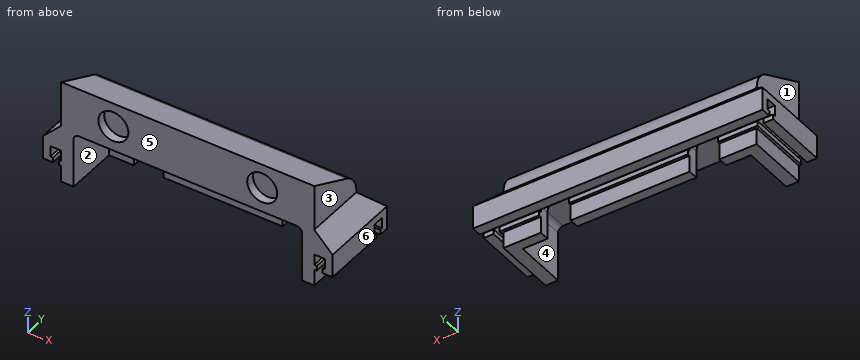
```python
from build123d import *

# Parameters (mm, degrees)
SKETCH1_W           = 102
SKETCH1_H           = 30
BOSS_EXTRUDE1_DEPTH = 25
CUT_EXTRUDE1_DEPTH  = 21
BOSS_EXTRUDE2_DEPTH = 102
SKETCH4_R           = 6.05
CUT_EXTRUDE2_DEPTH  = 3.5
FILLET1_R           = 10
CUT_EXTRUDE3_DEPTH  = 23.5
SKETCH6_W           = 1
SKETCH6_H           = 2
BOSS_EXTRUDE3_DEPTH = 25
SKETCH7_W           = 2
SKETCH7_H           = 1
BOSS_EXTRUDE4_DEPTH = 116.7
CUT_EXTRUDE4_DEPTH  = 7.35
SKETCH9_W           = 2.35
SKETCH9_H           = 1
SKETCH9_W_2         = 12
CUT_EXTRUDE5_DEPTH  = 3


with BuildPart() as part:
    # Sketch1 → Boss-Extrude1 (new body)
    with BuildSketch(Plane(origin=(0, 0, 0), x_dir=(1, 0, 0), z_dir=(0, 1, 0))):
        Rectangle(SKETCH1_W, SKETCH1_H)
    extrude(amount=BOSS_EXTRUDE1_DEPTH)

    # Sketch2 → Cut-Extrude1 (cut)
    with BuildSketch(Plane.XZ):
        with BuildLine():
            Line((-46, -37), (46, -37))
            Line((46, -37), (46, 5))
            ThreePointArc((46, 5), (45.414213562, 6.414213562), (44, 7))
            Line((44, 7), (-44, 7))
            ThreePointArc((-44, 7), (-45.414213562, 6.414213562), (-46, 5))
            Line((-46, 5), (-46, -37))
        make_face()
    extrude(amount=-CUT_EXTRUDE1_DEPTH, mode=Mode.SUBTRACT)

    # Sketch3 → Boss-Extrude2 (add)
    with BuildSketch(Plane(origin=(51, 0, 0), x_dir=(0, 0, -1), z_dir=(1, 0, 0))):
        Polygon((-15, 25), (-26.657691454, 0), (-15, 0), align=None)
    extrude(amount=-BOSS_EXTRUDE2_DEPTH)

    # Sketch4 → Cut-Extrude2 (cut)
    with BuildSketch(Plane.XZ):
        with Locations(Location((-30, 17, 0), (0, 0, 270))):
            Circle(SKETCH4_R)
        with Locations(Location((30, 17, 0), (0, 0, 270))):
            Circle(SKETCH4_R)
    extrude(amount=-CUT_EXTRUDE2_DEPTH, mode=Mode.SUBTRACT)

    # Fillet1
    fillet1_edges = [part.edges().sort_by_distance(p)[0] for p in [
        (0, 25, 15),
    ]]
    fillet(fillet1_edges, radius=FILLET1_R)

    # Sketch5 → Cut-Extrude3 (cut)
    with BuildSketch(Plane(origin=(0, 25, 0), x_dir=(1, 0, 0), z_dir=(0, 1, 0))):
        with BuildLine():
            Line((-24, 26), (-24, 4))
            ThreePointArc((-24, 4), (-30, -2), (-36, 4))
            Line((-36, 4), (-36, 26))
            ThreePointArc((-36, 26), (-30, 32), (-24, 26))
        make_face()
        with BuildLine():
            Line((24, 4), (24, 26))
            ThreePointArc((24, 26), (30, 32), (36, 26))
            Line((36, 26), (36, 4))
            ThreePointArc((36, 4), (30, -2), (24, 4))
        make_face()
    extrude(amount=-CUT_EXTRUDE3_DEPTH, mode=Mode.SUBTRACT)

    # Sketch6 → Boss-Extrude3 (add)
    with BuildSketch(Plane.XZ):
        Polygon((51, -2), (55.35, -2), (55.35, -6.35), (54.35, -6.35), (54.35, -8.35), (58.35, -8.35), (58.35, 1), (51, 8.35), align=None)
        with Locations((51.5, -7.35)):
            Rectangle(SKETCH6_W, SKETCH6_H)
    boss_extrude3 = extrude(amount=-BOSS_EXTRUDE3_DEPTH)

    # Sketch7 → Boss-Extrude4 (add)
    with BuildSketch(Plane(origin=(58.35, 0, 0), x_dir=(0, 0, -1), z_dir=(1, 0, 0))):
        Polygon((2, 25), (2, 29.35), (6.35, 29.35), (6.35, 28.35), (8.35, 28.35), (8.35, 32.35), (-1, 32.35), (-8.35, 25), align=None)
        with Locations((7.35, 25.5)):
            Rectangle(SKETCH7_W, SKETCH7_H)
    extrude(amount=-BOSS_EXTRUDE4_DEPTH)

    # Sketch8 → Cut-Extrude4 (cut)
    with BuildSketch(Plane.XZ.offset(-25)):
        Polygon((58.35, 8.35), (51, 8.35), (58.35, 1), align=None)
    cut_extrude4 = extrude(amount=-CUT_EXTRUDE4_DEPTH, mode=Mode.SUBTRACT)

    # Mirror1: Boss-Extrude3, Cut-Extrude4 across plane
    add(boss_extrude3.mirror(Plane(origin=(0, 0, 0), x_dir=(0, 0, 1), z_dir=(1, 0, 0))))
    add(cut_extrude4.mirror(Plane(origin=(0, 0, 0), x_dir=(0, 0, 1), z_dir=(1, 0, 0))), mode=Mode.SUBTRACT)

    # Sketch9 → Cut-Extrude5 (cut)
    with BuildSketch(Plane(origin=(0, 0, -8.35), x_dir=(-1, 0, 0), z_dir=(0, 0, -1))):
        with Locations((-53.175, 25.5)):
            Rectangle(SKETCH9_W, SKETCH9_H)
        with Locations((-30, 25.5)):
            Rectangle(SKETCH9_W_2, SKETCH9_H)
        with Locations((53.175, 25.5)):
            Rectangle(SKETCH9_W, SKETCH9_H)
        with Locations((30, 25.5)):
            Rectangle(SKETCH9_W_2, SKETCH9_H)
    extrude(amount=-CUT_EXTRUDE5_DEPTH, mode=Mode.SUBTRACT)


solid = part.part
```
Check sheet for the modelled part. Datum: model origin and axes. Units: mm. Face numbers are marked on the shaded views. A direction names the side the tool comes from. Coordinates: 2 decimals unless noted, no trailing zeros. Write each loop counter-clockwise with the first axis right and the second up, starting at its lowest first coordinate (ties: lowest second). Pieces come first, ordered by that corner, then holes. Notation, with made-up numbers: M 48,68 L 64,68 A25 cw 64,100 Z; hole C -25.5,42 d3. An arc over 180 degrees is marked long. Write item = value, one per line. Start each with the question number.
1. Tool access check on the marked faces 1, 2 and 3. Record the directions out of +Z, -Z, +X, -X, +Y, -Y that give a thin tool (end or side, any length) a straight path to the whole face; none if there is none.
2. Go/stop test with flat-tipped pins: pin 1 (5 mm diameter, centred on y = 21, z = 1.5, fed in from +X); pin 2 (1 mm diameter, centred on y = 28.5, z = 7.5, fed in from +X); pin 3 (10 mm diameter, centred on y = 5, z = 8.5, fed in from +X); pin 4 (0.5 mm diameter, centred on x = 11, y = 29, fed in from +Z). Record where each tip stops, or that it passes through.
3. Mould release check, pull along X, two halves, no side actions. Record for the marked faces 4, 5 and 6: pulls with the +X half, pulls with the -X half, needs draft (parallel to the pull), parting line crosses it, or undercut.
4. Sectioned sample at C-C (x = -30). Record the cut outline in (y, z).
5. Sectioned sample at A-A (x = 2). Record the cut outline in (y, z).
6. Thickness scan on probe 1 along X at (y, z) = (1, 17); probe 2 along X at (y, z) = (1.5, -2.5); probe 3 along X at (y, z) = (16, -1). Record the ranges inside material, lowest first.
The answers:
q1.face_1 = +Z, -X, +Y, -Y
q1.face_2 = -Z, -Y
q1.face_3 = +Z, +X, +Y, -Y
q2.pin_1 = 58.35
q2.pin_2 = through
q2.pin_3 = 55.85
q2.pin_4 = 4.6
q3.face_4 = undercut
q3.face_5 = needs draft
q3.face_6 = pulls with the +X half
q4.outline = M 0,7 L 21,7 L 21,2 L 25,2 L 25,-2 L 29.35,-2 L 29.35,-6.35 L 28.35,-6.35 L 28.35,-8.35 L 32.35,-8.35 L 32.35,1 L 25,8.35 L 25,8.63 A10 ccw 19.23,17.69 L 0,26.66 L 0,23.05 L 3.5,23.05 L 3.5,10.95 L 0,10.95 Z
q5.outline = M 0,7 L 21,7 L 21,-15 L 25,-15 L 25,-8.35 L 26,-8.35 L 26,-6.35 L 25,-6.35 L 25,-2 L 29.35,-2 L 29.35,-6.35 L 28.35,-6.35 L 28.35,-8.35 L 32.35,-8.35 L 32.35,1 L 25,8.35 L 25,8.63 A10 ccw 19.23,17.69 L 0,26.66 Z
q6.probe_1 = -51 to -36.05, -23.95 to 23.95, 36.05 to 51
q6.probe_2 = -58.35 to -55.35, -51 to -46, 46 to 51, 55.35 to 58.35
q6.probe_3 = -58.35 to -46, 46 to 58.35
